Check sheet for the modelled part. Datum: model origin and axes. Units: mm. Give positions to 0.01 mm unless a question says otherwise; leave off trailing zeros. Order: outer loops, then holes, each group sorted by start corner. A loop starts at its lowest first (then second) coordinate and runs counter-clockwise, first axis right, second up.
Item 1: Gauge pin test, flat ends, axial feed: P1, Ø3, axis at x = 53.5, z = 44, coming from the +Y side; P2, Ø2, axis at y = 2, z = -5, coming from the -X side; P3, Ø4, axis at x = -54.5, z = 62, coming from the +Y side; P4, Ø8, axis at x = 54.5, z = -62, coming from the -Y side. Record the tip position at first contact, or that the pin passes through.
Item 2: Material ranges on line 1 along X through (y, z) = (1.1, 24.35); line 2 along X through (y, z) = (-5.5, 39.5); line 3 along X through (y, z) = (1.3, 62), recorded low to high.
Item 3: Sectioned sample at A-A on y = -4. Count the separate pieces of the cut face and the enclosed holes in it, and give its area (3 significant figures).
Item 4: Sectioned sample at D-D on x = 13. Record the boundary of the cut face in (y, z), and give its area (3 significant figures).
Item 5: Sectioned sample at C-C on z = -43.5. Record the boundary of the cut face in (x, y), and give its area (3 significant figures).
Item 6: Sectioned sample at B-B on z = 62. Record the boundary of the cut face in (x, y).
from build123d import *

# Parameters (mm, degrees)
SKETCH1_W           = 120
SKETCH1_H           = 140
BOSS_EXTRUDE1_DEPTH = 4
SKETCH2_W           = 12
SKETCH2_H           = 23
SKETCH2_H_2         = 34
SKETCH2_R           = 1.1
SKETCH2_R_2         = 2.5
CUT_EXTRUDE1_DEPTH  = 93.28217596
SKETCH3_W           = 2.5
SKETCH3_H           = 140
BOSS_EXTRUDE2_DEPTH = 4
SKETCH7_W           = 2.5
SKETCH7_H           = 10
BOSS_EXTRUDE6_DEPTH = 10
SKETCH8_W           = 17
SKETCH8_H           = 10
BOSS_EXTRUDE7_DEPTH = 2
SKETCH9_R           = 3.4
BOSS_EXTRUDE8_DEPTH = 2
SKETCH10_W          = 2.5
SKETCH10_H          = 34
CUT_EXTRUDE2_DEPTH  = 96.552341677
FILLET1_R           = 10
FILLET2_R           = 10
FILLET3_R           = 10
FILLET4_R           = 10
FILLET5_R           = 3
FILLET6_R           = 3
FILLET7_R           = 3
FILLET8_R           = 3


with BuildPart() as part:
    # Sketch1 → Boss-Extrude1 (new body)
    with BuildSketch(Plane(origin=(0, 0, 0), x_dir=(1, 0, 0), z_dir=(0, 1, 0))):
        Rectangle(SKETCH1_W, SKETCH1_H)
    extrude(amount=BOSS_EXTRUDE1_DEPTH)

    # Sketch2 → Cut-Extrude1 (cut, through all)
    with BuildSketch(Plane(origin=(0, 4, 0), x_dir=(1, 0, 0), z_dir=(0, 1, 0))):
        with Locations((54, 38.5)):
            Rectangle(SKETCH2_W, SKETCH2_H)
        with Locations((-54, 38.5)):
            Rectangle(SKETCH2_W, SKETCH2_H)
        with Locations((54, -38.5)):
            Rectangle(SKETCH2_W, SKETCH2_H)
        with Locations((-54, -38.5)):
            Rectangle(SKETCH2_W, SKETCH2_H)
        with Locations((-54, 0)):
            Rectangle(SKETCH2_W, SKETCH2_H_2)
        with Locations((54, 0)):
            Rectangle(SKETCH2_W, SKETCH2_H_2)
        with Locations(Location((-54, 52.65, 0), (0, 0, 270))):
            Circle(SKETCH2_R)
        with Locations(Location((-54, 24.35, 0), (0, 0, 270))):
            Circle(SKETCH2_R)
        with Locations(Location((-54, -24.35, 0), (0, 0, 270))):
            Circle(SKETCH2_R)
        with Locations(Location((-54, -52.65, 0), (0, 0, 270))):
            Circle(SKETCH2_R)
        with Locations(Location((54, 52.65, 0), (0, 0, 270))):
            Circle(SKETCH2_R)
        with Locations(Location((54, 24.35, 0), (0, 0, 270))):
            Circle(SKETCH2_R)
        with Locations(Location((54, -24.35, 0), (0, 0, 270))):
            Circle(SKETCH2_R)
        with Locations(Location((54, -52.65, 0), (0, 0, 270))):
            Circle(SKETCH2_R)
        with Locations(Location((-54.5, 62, 0), (0, 0, 270))):
            Circle(SKETCH2_R_2)
        with Locations(Location((54.5, 62, 0), (0, 0, 270))):
            Circle(SKETCH2_R_2)
        with Locations(Location((54.5, -62, 0), (0, 0, 270))):
            Circle(SKETCH2_R_2)
        with Locations(Location((-54.5, -62, 0), (0, 0, 270))):
            Circle(SKETCH2_R_2)
    extrude(amount=-CUT_EXTRUDE1_DEPTH, mode=Mode.SUBTRACT)

    # Sketch3 → Boss-Extrude2 (add)
    with BuildSketch(Plane(origin=(0, 4, 0), x_dir=(1, 0, 0), z_dir=(0, 1, 0))):
        with Locations((61.25, 0)):
            Rectangle(SKETCH3_W, SKETCH3_H)
        with Locations((-61.25, 0)):
            Rectangle(SKETCH3_W, SKETCH3_H)
    extrude(amount=-BOSS_EXTRUDE2_DEPTH)

    # Sketch7 → Boss-Extrude6 (add)
    with BuildSketch(Plane.XZ):
        with Locations((46.75, 43.5)):
            Rectangle(SKETCH7_W, SKETCH7_H)
        with Locations((61.25, 43.5)):
            Rectangle(SKETCH7_W, SKETCH7_H)
        with Locations((-61.25, 43.5)):
            Rectangle(SKETCH7_W, SKETCH7_H)
        with Locations((-46.75, 43.5)):
            Rectangle(SKETCH7_W, SKETCH7_H)
        with Locations((-61.25, -43.5)):
            Rectangle(SKETCH7_W, SKETCH7_H)
        with Locations((-46.75, -43.5)):
            Rectangle(SKETCH7_W, SKETCH7_H)
        with Locations((46.75, -43.5)):
            Rectangle(SKETCH7_W, SKETCH7_H)
        with Locations((61.25, -43.5)):
            Rectangle(SKETCH7_W, SKETCH7_H)
    extrude(amount=BOSS_EXTRUDE6_DEPTH)

    # Sketch8 → Boss-Extrude7 (add)
    with BuildSketch(Plane.XZ.offset(10)):
        with Locations((-54, 43.5)):
            Rectangle(SKETCH8_W, SKETCH8_H)
        with Locations((-54, -43.5)):
            Rectangle(SKETCH8_W, SKETCH8_H)
        with Locations((54, -43.5)):
            Rectangle(SKETCH8_W, SKETCH8_H)
        with Locations((54, 43.5)):
            Rectangle(SKETCH8_W, SKETCH8_H)
    extrude(amount=BOSS_EXTRUDE7_DEPTH)

    # Sketch9 → Boss-Extrude8 (add)
    with BuildSketch(Plane.XZ.offset(12)):
        with Locations(Location((54, 43.5, 0), (0, 0, 270))):
            Circle(SKETCH9_R)
        with Locations(Location((-54, 43.5, 0), (0, 0, 270))):
            Circle(SKETCH9_R)
        with Locations(Location((-54, -43.5, 0), (0, 0, 270))):
            Circle(SKETCH9_R)
        with Locations(Location((54, -43.5, 0), (0, 0, 270))):
            Circle(SKETCH9_R)
    extrude(amount=BOSS_EXTRUDE8_DEPTH)

    # Sketch10 → Cut-Extrude2 (cut, through all)
    with BuildSketch(Plane(origin=(0, 4, 0), x_dir=(1, 0, 0), z_dir=(0, 1, 0))):
        with Locations((61.25, 0)):
            Rectangle(SKETCH10_W, SKETCH10_H)
        with Locations((-61.25, 0)):
            Rectangle(SKETCH10_W, SKETCH10_H)
    extrude(amount=-CUT_EXTRUDE2_DEPTH, mode=Mode.SUBTRACT)

    # Fillet1
    fillet1_edges = [part.edges().sort_by_distance(p)[0] for p in [
        (62.5, 2, -70),
    ]]
    fillet(fillet1_edges, radius=FILLET1_R)

    # Fillet2
    fillet2_edges = [part.edges().sort_by_distance(p)[0] for p in [
        (-62.5, 2, -70),
    ]]
    fillet(fillet2_edges, radius=FILLET2_R)

    # Fillet3
    fillet3_edges = [part.edges().sort_by_distance(p)[0] for p in [
        (-62.5, 2, 70),
    ]]
    fillet(fillet3_edges, radius=FILLET3_R)

    # Fillet4
    fillet4_edges = [part.edges().sort_by_distance(p)[0] for p in [
        (62.5, 2, 70),
    ]]
    fillet(fillet4_edges, radius=FILLET4_R)

    # Fillet5
    fillet5_edges = [part.edges().sort_by_distance(p)[0] for p in [
        (62.5, 2, -17),
    ]]
    fillet(fillet5_edges, radius=FILLET5_R)

    # Fillet6
    fillet6_edges = [part.edges().sort_by_distance(p)[0] for p in [
        (-62.5, 2, 17),
    ]]
    fillet(fillet6_edges, radius=FILLET6_R)

    # Fillet7
    fillet7_edges = [part.edges().sort_by_distance(p)[0] for p in [
        (62.5, 2, 17),
    ]]
    fillet(fillet7_edges, radius=FILLET7_R)

    # Fillet8
    fillet8_edges = [part.edges().sort_by_distance(p)[0] for p in [
        (-62.5, 2, -17),
    ]]
    fillet(fillet8_edges, radius=FILLET8_R)


solid = part.part
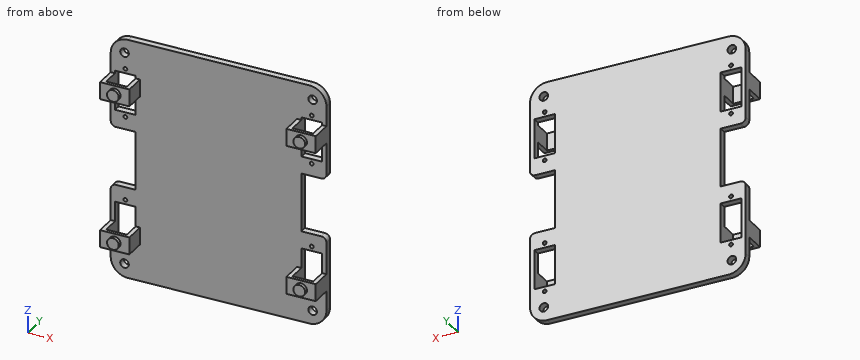
Report:
1. P1: stops at y = -10
1. P2: stops at x = -48
1. P3: passes through
1. P4: stops at y = 0
2. line 1: x = -62.5 to -55.1, -52.9 to 52.9, 55.1 to 62.5
2. line 2: x = -62.5 to -60, -48 to -45.5, 45.5 to 48, 60 to 62.5
2. line 3: x = -62.3 to -57, -52 to 52, 57 to 62.3
3. separate pieces: 8
3. enclosed holes: 0
3. area: 200 mm2
4. outline: (0, -70) - (4, -70) - (4, 70) - (0, 70) - close
4. area: 560 mm2
5. outline: (-62.5, -12) - (-57.4, -12) - (-57.4, -14) - (-50.6, -14) - (-50.6, -12) - (-45.5, -12) - (-45.5, 0) - (45.5, 0) - (45.5, -12) - (50.6, -12) - (50.6, -14) - (57.4, -14) - (57.4, -12) - (62.5, -12) - (62.5, 4) - (60, 4) - (60, -10) - (48, -10) - (48, 4) - (-48, 4) - (-48, -10) - (-60, -10) - (-60, 4) - (-62.5, 4) - close
5. area: 599 mm2
6. outline: (-62.3, 0) - (-57, 0) - (-57, 4) - (-62.3, 4) - close; (-52, 0) - (52, 0) - (52, 4) - (-52, 4) - close; (57, 0) - (62.3, 0) - (62.3, 4) - (57, 4) - close
